```python
from build123d import *

# Parameters (mm, degrees)
F0_W     = 25.4
F0_H     = 25.4
F0_W_2   = 19.05
F0_H_2   = 19.05
F1_DEPTH = 495.3
F2_R     = 9.525
F3_DEPTH = 25.4
F4_R     = 9.525
F5_DEPTH = 25.4


with BuildPart() as f1:
    # F0 (on Top) → F1 (new body)
    with BuildSketch(Plane.XY):
        Rectangle(F0_W, F0_H)
        Rectangle(F0_W_2, F0_H_2, mode=Mode.SUBTRACT)
    extrude(amount=F1_DEPTH)

    # F2 (on face) → F3 (cut)
    with BuildSketch(Plane.YZ.offset(12.7)):
        with Locations((0, 469.9)):
            Circle(F2_R)
    extrude(amount=-F3_DEPTH, mode=Mode.SUBTRACT)

    # F4 (on face) → F5 (cut)
    with BuildSketch(Plane.YZ.offset(12.7)):
        with Locations((0, 12.7)):
            Circle(F4_R)
    extrude(amount=-F5_DEPTH, mode=Mode.SUBTRACT)


solid = f1.part
```
Could you check a few things on this model? Use its own coordinates, in mm. A direction names the side the tool comes from. Coordinates: 2 decimals unless noted, no trailing zeros. Order: outer loops, then holes, each group sorted by start corner. A loop starts at its lowest first (then second) coordinate and runs counter-clockwise, first axis right, second up. Notation, with made-up numbers: M 32,15.5 L 51,15.5 A11 ccw 51,19.5 Z; hole C -20.5,-34.75 d11. An arc over 180 degrees is marked long. Use a Markdown table: item, result. Add a question column.
Q1. I want a section at B-B on z = 430. List the corners of the cut face in (x, y) for me (3 decimals), then the cut area to 3 significant figures.
Q2. Which directions (+Z, -Z, +X, -X, +Y, -Y) give clear straight access to the entire face, cutting with the end or side of a thin tool? Please do faces 4 (the flat face through (9.525, 0, 485)), 5 (the flat face through (0, -12.7, 244)).
Q3. We'd pull the mould along Z, two halves only. Please class faces 1 (the cylindrical face through (-11.09, -2.06, 460.6)), 2 (the flat face through (11, 0, 0)), 3 (the flat face through (-9.525, 0, 2)): pulls with the +Z half, pulls with the -Z half, needs draft (parallel to the pull), parting line crosses it, or undercut.
Q4. I want a section at C-C on x = -2. List the corners of the cut face in (y, z) for me (3 decimals), then the cut area to 3 significant figures.
Q5. If I drill on L1, parallel to Z at x = 11.45, y = 0 (3 decimals); L2, parallel to Y at x = -0.5, z = 46.5 (3 decimals), over which ranges is the centre line in solid material (lowest first)?
Q6. I want a section at A-A on y = 0. List the corners of the cut face in (x, z) for me (3 decimals), then the cut area to 3 significant figures.
Checked values:
| question | item | result |
|---|---|---|
| 1 | outline | M -12.7,-12.7 L 12.7,-12.7 L 12.7,12.7 L -12.7,12.7 Z; hole M -9.525,-9.525 L 9.525,-9.525 L 9.525,9.525 L -9.525,9.525 Z |
| 1 | area | 282 mm² |
| 2 | face 4 | +Z, -Z |
| 2 | face 5 | +Z, -Z, +X, -X, -Y |
| 3 | face 1 | undercut |
| 3 | face 2 | pulls with the -Z half |
| 3 | face 3 | needs draft |
| 4 | outline | M -12.7,0 L -9.525,0 L -9.525,495.3 L -12.7,495.3 Z; M 9.525,0 L 12.7,0 L 12.7,495.3 L 9.525,495.3 Z |
| 4 | area | 3,150 mm² |
| 5 | L1 | 0 to 3.175, 22.225 to 460.375, 479.425 to 495.3 |
| 5 | L2 | -12.7 to -9.525, 9.525 to 12.7 |
| 6 | outline | M -12.7,0 L -9.525,0 L -9.525,3.175 L -12.7,3.175 Z; M -12.7,22.225 L -9.525,22.225 L -9.525,460.375 L -12.7,460.375 Z; M -12.7,479.425 L -9.525,479.425 L -9.525,495.3 L -12.7,495.3 Z; M 9.525,0 L 12.7,0 L 12.7,3.175 L 9.525,3.175 Z; M 9.525,22.225 L 12.7,22.225 L 12.7,460.375 L 9.525,460.375 Z; M 9.525,479.425 L 12.7,479.425 L 12.7,495.3 L 9.525,495.3 Z |
| 6 | area | 2,900 mm² |
